from build123d import *

# Parameters (mm, degrees)
ESBO_O1_W                = 140
ESBO_O1_H                = 140
ESBO_O1_R                = 2.5
RESSALTO_EXTRUS_O1_DEPTH = 10
ESBO_O2_R                = 7
ESBO_O2_R_2              = 2.5
RESSALTO_EXTRUS_O2_DEPTH = 24
FILETE1_R                = 10
FILETE2_R                = 10
FILETE3_R                = 10
FILETE4_R                = 10
FILETE5_R                = 10


with BuildPart() as part:
    # Esboço1 → Ressalto-extrusão1 (new body)
    with BuildSketch(Plane.XY):
        with Locations((34.130618452, 70)):
            Rectangle(ESBO_O1_W, ESBO_O1_H)
        with Locations((34.130618452, 70)):
            Circle(ESBO_O1_R, mode=Mode.SUBTRACT)
    extrude(amount=RESSALTO_EXTRUS_O1_DEPTH)

    # Esboço2 → Ressalto-extrusão2 (add)
    with BuildSketch(Plane.XY):
        with Locations(Location((34.130618452, 70, 0), (0, 0, 180))):
            Circle(ESBO_O2_R)
        with Locations((34.130618452, 70)):
            Circle(ESBO_O2_R_2, mode=Mode.SUBTRACT)
    extrude(amount=RESSALTO_EXTRUS_O2_DEPTH)

    # Filete1
    filete1_edges = [part.edges().sort_by_distance(p)[0] for p in [
        (34.130618452, 0, 10),
    ]]
    fillet(filete1_edges, radius=FILETE1_R - 0.0001)  # a hair under: the kernel refuses the full size

    # Filete2
    filete2_edges = [part.edges().sort_by_distance(p)[0] for p in [
        (34.130618452, 140, 10),
    ]]
    fillet(filete2_edges, radius=FILETE2_R - 0.0001)  # a hair under: the kernel refuses the full size

    # Filete3
    filete3_edges = [part.edges().sort_by_distance(p)[0] for p in [
        (-35.869381548, 2.928902899, 7.071097101),
        (-35.869381548, 70, 10),
        (-35.869381548, 137.071097101, 7.071097101),
    ]]
    fillet(filete3_edges, radius=FILETE3_R - 0.0001)  # a hair under: the kernel refuses the full size

    # Filete4
    filete4_edges = [part.edges().sort_by_distance(p)[0] for p in [
        (104.130618452, 70, 10),
        (104.130618452, 2.928902899, 7.071097101),
        (104.130618452, 137.071097101, 7.071097101),
    ]]
    fillet(filete4_edges, radius=FILETE4_R - 0.0001)  # a hair under: the kernel refuses the full size

    # Filete5
    filete5_edges = [part.edges().sort_by_distance(p)[0] for p in [
        (41.130618452, 70, 10),
    ]]
    fillet(filete5_edges, radius=FILETE5_R)


solid = part.part
Build history of the part. All positions in model axes, mm. A direction names the side the tool comes from. Give positions to 0.01 mm unless a question says otherwise; leave off trailing zeros. Loops run counter-clockwise (first coordinate to the right, second up) from the corner with the lowest first, then second, coordinate; pieces in that order, holes last. Notation, with made-up numbers: (-15.75, 50.25) -> (32.25, 50.25) arc R22 ccw to (32.25, 65.25) -> close; hole circle Ø3 at (-28.5, 81.5). An arc over 180 degrees is marked (long way). Answer in a Markdown table with one row per item.
Item 1: Slice it at B-B on z = 4. Write the cut outline in (x, y).
Findings below:
| item | result |
|---|---|
| outline | (-35.03, 10) arc R9.17 ccw to (-25.87, 0.83) -> (94.13, 0.83) arc R9.17 ccw to (103.3, 10) -> (103.3, 130) arc R9.17 ccw to (94.13, 139.17) -> (-25.87, 139.17) arc R9.17 ccw to (-35.03, 130) -> close; hole circle Ø5 at (34.13, 70) |
Item 2: Probe line 1 along Z through (x, y) = (5.5, 89.5); line 2 along Y through (x, z) = (60, 5); line 3 along Y through (x, z) = (10.5, 2.75). List the from-to ranges inside material, lowest first. Write a range as [from, to].
Findings below:
| item | result |
|---|---|
| line 1 | z = [0, 10] |
| line 2 | y = [1.34, 138.66] |
| line 3 | y = [0.39, 139.61] |
Item 3: Mould opens along Y. For faces 1 (the flat face through (18, 71, 0)), 2 (the cylindrical face through (34.97, 136.99, 7.15)), 3 (the cylindrical face through (32.147, 68.479, 11.832)) say: pulls with the +Y half, pulls with the -Y half, needs draft (parallel to the pull), parting line crosses it, or undercut.
Findings below:
| item | result |
|---|---|
| face 1 | needs draft |
| face 2 | pulls with the +Y half |
| face 3 | undercut |
Item 4: Tool access for faces 4 (the cylindrical face through (35.04, 63.06, 21.97)), 5 (the flat face through (31, 70, 24)): list every direction of +Z, -Z, +X, -X, +Y, -Y with a clear straight run to the whole face (end or side of a thin tool).
Findings below:
| item | result |
|---|---|
| face 4 | +Z |
| face 5 | +Z, +X, -X, +Y, -Y |
Item 5: Flat gauge pins, fed straight in: P1, Ø10, axis at y = 68.5, z = 7.5, coming from the +X side; P2, Ø6, axis at y = 124, z = 8.5, coming from the +X side; P3, Ø4, axis at y = 60.5, z = 4.5, coming from the -X side. Where does each tip first touch, or does it go through?
Findings below:
| item | result |
|---|---|
| P1 | stops at x = 103.81 |
| P2 | stops at x = 102.48 |
| P3 | stops at x = -35.55 |
